The model under review builds one solid part; all positions refer to its coordinate system, in mm. Face numbers are marked on the shaded views. A direction names the side the tool comes from. Give positions to 0.01 mm unless a question says otherwise; leave off trailing zeros. Write each loop counter-clockwise with the first axis right and the second up, starting at its lowest first coordinate (ties: lowest second). Pieces come first, ordered by that corner, then holes. Notation, with made-up numbers: (-6.75, 77.25) -> (9.25, 77.25) arc R14 cw to (9.25, 101.25) -> close; hole circle Ø1 at (0, 31). An arc over 180 degrees is marked (long way). Use CSV: the item, a comma, the result in double quotes.
```python
from build123d import *

# Parameters (mm, degrees)
PAD_DEPTH       = 80
SKETCH001_R     = 1.5
HOLE_DEPTH      = 25
HOLE_TIPS_R     = 1.5
SKETCH002_R     = 1.5
HOLE001_DEPTH   = 25
SKETCH003_W     = 17.76
SKETCH003_H     = 43.16
POCKET_DEPTH    = 3
SKETCH004_W     = 9
SKETCH004_H     = 9
POCKET001_DEPTH = 3


with BuildPart() as part:
    # Sketch → Pad (new body)
    with BuildSketch(Plane.XZ):
        Polygon((-125, 0), (125, 0), (125, 15), (38.06, 15), (12.5, 35.873102), (12.5, 140.603102), (-12.5, 140.603102), (-12.5, 35.873102), (-38.06, 15), (-125, 15), align=None)
    extrude(amount=PAD_DEPTH)

    # Sketch001 (on Face5 of Pad) → Hole (cut)
    with BuildSketch(Plane(origin=(12.5, 0, 0), x_dir=(0, 0, 1), z_dir=(1, 0, 0))):
        with Locations((135.603102, 63)):
            Circle(SKETCH001_R)
        with Locations((135.603102, 17)):
            Circle(SKETCH001_R)
    extrude(amount=-HOLE_DEPTH, mode=Mode.SUBTRACT)

    # Hole tips → Hole tip 1 section 0
    with BuildSketch(Plane(origin=(-12.5, 0, 0), x_dir=(0, 0, 1), z_dir=(1, 0, 0)), mode=Mode.PRIVATE) as hole_tip_1_s0:
        with Locations((135.603102, 63)):
            Circle(HOLE_TIPS_R)
    loft([hole_tip_1_s0.sketch, Vertex(-13.401291, -63, 135.603102)], mode=Mode.SUBTRACT)

    # Hole tips → Hole tip 2 section 0
    with BuildSketch(Plane(origin=(-12.5, 0, 0), x_dir=(0, 0, 1), z_dir=(1, 0, 0)), mode=Mode.PRIVATE) as hole_tip_2_s0:
        with Locations((135.603102, 17)):
            Circle(HOLE_TIPS_R)
    loft([hole_tip_2_s0.sketch, Vertex(-13.401291, -17, 135.603102)], mode=Mode.SUBTRACT)

    # Sketch002 (on Face7 of Hole) → Hole001 (cut)
    with BuildSketch(Plane(origin=(0, 0, 15), x_dir=(-1, 0, 0), z_dir=(0, 0, 1))):
        with Locations((53.06, 62.5)):
            Circle(SKETCH002_R)
        with Locations((73.06, 62.5)):
            Circle(SKETCH002_R)
        with Locations((53.06, 17.5)):
            Circle(SKETCH002_R)
        with Locations((73.06, 17.5)):
            Circle(SKETCH002_R)
    extrude(amount=-HOLE001_DEPTH, mode=Mode.SUBTRACT)

    # Sketch003 (on Face10 of Hole001) → Pocket (cut)
    with BuildSketch(Plane(origin=(0, 0, 15), x_dir=(-1, 0, 0), z_dir=(0, 0, 1))):
        with Locations((91.94, 40)):
            Rectangle(SKETCH003_W, SKETCH003_H)
    extrude(amount=-POCKET_DEPTH, mode=Mode.SUBTRACT)

    # Sketch004 (on Face10 of Pocket) → Pocket001 (cut)
    with BuildSketch(Plane(origin=(0, 0, 15), x_dir=(-1, 0, 0), z_dir=(0, 0, 1))):
        with Locations((91.94, 66.08)):
            Rectangle(SKETCH004_W, SKETCH004_H)
        with Locations((91.94, 13.92)):
            Rectangle(SKETCH004_W, SKETCH004_H)
    extrude(amount=-POCKET001_DEPTH, mode=Mode.SUBTRACT)


solid = part.part
```
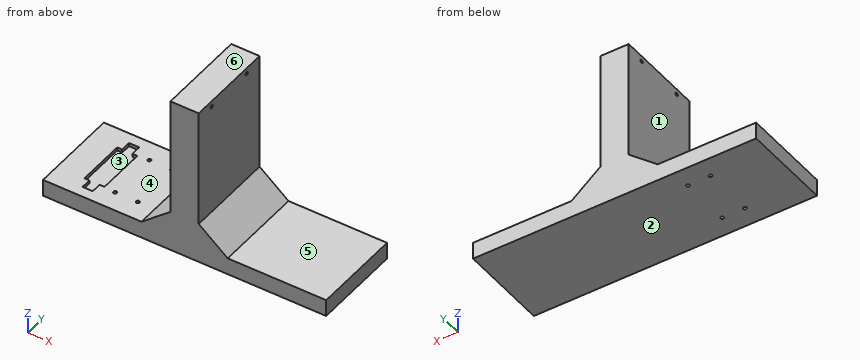
Q1. Insertion check: pin 1 (1.5 mm diameter, centred on x = -48.5, y = -12, fed in from +Z); pin 2 (14 mm diameter, centred on x = -91, y = -37, fed in from +Z); pin 3 (1.5 mm diameter, centred on x = 24, y = -52.5, fed in from +Z); pin 4 (2.5 mm diameter, centred on x = -92, z = 13.5, fed in from +Y). Each pin has a flat end and moves straight along its axis. Give the tip position at first contact, or say it passes through.
Derived:
pin 1,"stops at z = 15"
pin 2,"stops at z = 12"
pin 3,"stops at z = 27.09"
pin 4,"stops at y = 0"
Q2. Consider section A-A (y = -12.5). Write out the cut boundary in (x, z), then the cut area to 3 significant figures.
Derived:
outline,"(-125, 0) -> (125, 0) -> (125, 15) -> (38.06, 15) -> (12.5, 35.87) -> (12.5, 140.6) -> (-12.5, 140.6) -> (-12.5, 35.87) -> (-38.06, 15) -> (-87.44, 15) -> (-87.44, 12) -> (-96.44, 12) -> (-96.44, 15) -> (-125, 15) -> close"
area,"7,400 mm2"
Q3. To check wall thickness, follow probe 1 along Y at (x, z) = (-53, 9); probe 2 along X at (y, z) = (-17.5, 3.5); probe 3 along X at (y, z) = (-66, 120.5). State the ranges of each line that lie inside material, in increasing order.
Derived:
probe 1,"y = -80 to -64, -61 to -19, -16 to 0"
probe 2,"x = -125 to -74.56, -71.56 to -54.56, -51.56 to 125"
probe 3,"x = -12.5 to 12.5"
Q4. Machinability: for the marked faces 4, 5 and 6, which of the approach directions +Z, -Z, +X, -X, +Y, -Y give a long, thin tool a straight path to every point of the face, cutting with its end or side? Answer none if there is none.
Derived:
face 4,"+Z, -X, +Y, -Y"
face 5,"+Z, +X, +Y, -Y"
face 6,"+Z, +X, -X, +Y, -Y"
Q5. Consider section D-D (y = -41.5). Write out the cut boundary in (x, z), then the cut area to 3 significant figures.
Derived:
outline,"(-125, 0) -> (125, 0) -> (125, 15) -> (38.06, 15) -> (12.5, 35.87) -> (12.5, 140.6) -> (-12.5, 140.6) -> (-12.5, 35.87) -> (-38.06, 15) -> (-83.06, 15) -> (-83.06, 12) -> (-100.82, 12) -> (-100.82, 15) -> (-125, 15) -> close"
area,"7,370 mm2"
Q6. Consider section B-B (x = -40.5). Write out the cut boundary in (y, z).
Derived:
outline,"(-80, 0) -> (0, 0) -> (0, 15) -> (-80, 15) -> close"
Q7. The part is to be moulded in two halves that separate along X. For the marked faces 1, 2 and 3, say which applies: pulls with the +X half, pulls with the -X half, needs draft (parallel to the pull), parting line crosses it, or undercut.
Derived:
face 1,"pulls with the -X half"
face 2,"needs draft"
face 3,"undercut"
Q8. Consider section C-C (z = 52.5). Write out the cut boundary in (x, y), then the cut area to 3 significant figures.
Derived:
outline,"(-12.5, -80) -> (12.5, -80) -> (12.5, 0) -> (-12.5, 0) -> close"
area,"2,000 mm2"
